Input: part model. Units: mm. Frame: model coordinates. A direction names the side the tool comes from. Give positions to 0.01 mm unless a question says otherwise; leave off trailing zeros. Order: outer loops, then holes, each group sorted by start corner. A loop starts at its lowest first (then second) coordinate and runs counter-clockwise, first axis right, second up. Notation, with made-up numbers: (-15, 44) -> (41, 44) arc R12 cw to (41, 66) -> close; hole circle Ø11 at (-38, 32). An arc over 180 degrees is marked (long way). Use a Markdown table: item, result. Add a question column.
from build123d import *

# Parameters (mm, degrees)
F1_DEPTH      = 25.4
F2_DEPTH      = 20.32
F3_SIZE2      = 12.7
F3_SIZE       = 25.4
F4_SIZE2      = 25.4
F4_SIZE       = 12.7
F4_2_SIZE2    = 25.4
F4_2_SIZE     = 12.7
F5_R          = 16.1148296274
F6_DEPTH      = 103.886
F8_DEPTH      = 109.4047297446
F8_DEPTH_BACK = 116.5023496438
F9_R          = 3.3795298113
F10_DEPTH     = 138.2457237613


with BuildPart() as f1:
    # F0 (on Top) → F1 (new body)
    with BuildSketch(Plane.XY):
        with BuildLine():
            ThreePointArc((52.5300336642, -32.2163809765), (59.3056389857, -16.7374079377), (61.6222333252, 0))
            ThreePointArc((61.6222333252, 0), (49.8558080108, 36.2173721792), (19.05, 58.6037297446))
            ThreePointArc((19.05, 58.6037297446), (0, 61.6222333252), (-19.05, 58.6037297446))
            ThreePointArc((-19.05, 58.6037297446), (-57.8186685482, 21.31434276), (-52.5300336642, -32.2163809765))
            ThreePointArc((-52.5300336642, -32.2163809765), (-39.9894732611, -46.8843435305), (-23.5270019404, -56.9541905366))
            ThreePointArc((-23.5270019404, -56.9541905366), (0, -61.6222333252), (23.5270019404, -56.9541905366))
            ThreePointArc((23.5270019404, -56.9541905366), (39.9894732611, -46.8843435305), (52.5300336642, -32.2163809765))
        make_face()
    extrude(amount=F1_DEPTH)

    # F0 (on Top) → F2 (join)
    with BuildSketch(Plane.XY):
        with BuildLine():
            ThreePointArc((-23.5270019404, -56.9541905366), (-39.9894732611, -46.8843435305), (-52.5300336642, -32.2163809765))
            Line((-52.5300336642, -32.2163809765), (-100.8460948708, -92.7285929554))
            Line((-100.8460948708, -92.7285929554), (-71.0725153171, -116.5013496438))
            Line((-71.0725153171, -116.5013496438), (-23.5270019404, -56.9541905366))
        make_face()
        with BuildLine():
            ThreePointArc((-19.05, 58.6037297446), (0, 61.6222333252), (19.05, 58.6037297446))
            Line((19.05, 58.6037297446), (19.05, 109.4037297446))
            Line((19.05, 109.4037297446), (-19.05, 109.4037297446))
            Line((-19.05, 109.4037297446), (-19.05, 58.6037297446))
        make_face()
        with BuildLine():
            Line((100.8460948708, -92.7285929554), (52.5300336642, -32.2163809765))
            ThreePointArc((52.5300336642, -32.2163809765), (39.9894732611, -46.8843435305), (23.5270019404, -56.9541905366))
            Line((23.5270019404, -56.9541905366), (71.0725153171, -116.5013496438))
            Line((71.0725153171, -116.5013496438), (100.8460948708, -92.7285929554))
        make_face()
    extrude(amount=F2_DEPTH)

    # F3
    f3_edges = [f1.edges().sort_by_distance(p)[0] for p in [
        (85.959305, -104.614971, 20.32),
    ]]
    f3_side = f1.faces().sort_by_distance((62.662137, -75.354715, 20.32))[0]
    chamfer(f3_edges, length=F3_SIZE, length2=F3_SIZE2, reference=f3_side)

    # F4
    f4_edges = [f1.edges().sort_by_distance(p)[0] for p in [
        (-85.959305, -104.614971, 20.32),
    ]]
    f4_side = f1.faces().sort_by_distance((-85.959305, -104.614971, 10.16))[0]
    chamfer(f4_edges, length=F4_SIZE, length2=F4_SIZE2, reference=f4_side)

    # F4#2
    f4_2_edges = [f1.edges().sort_by_distance(p)[0] for p in [
        (0, 109.40373, 20.32),
    ]]
    f4_2_side = f1.faces().sort_by_distance((0, 109.40373, 10.16))[0]
    chamfer(f4_2_edges, length=F4_2_SIZE, length2=F4_2_SIZE2, reference=f4_2_side)

    # F5 (on face) → F6 (join)
    with BuildSketch(Plane.XY.offset(25.4)):
        with Locations((-30.9876389802, 0)):
            Circle(F5_R)
        with Locations((30.9876389802, 0)):
            Circle(F5_R)
    extrude(amount=F6_DEPTH)

    # F7 (on Front) → F8 (cut, two sides)
    with BuildSketch(Plane.XZ) as f8_sk:
        Polygon((47.1024686075, 129.286), (37.3986288905, 129.286), (37.3986288905, 99.2526204783), (47.1024686075, 93.5718588345), align=None)
        Polygon((-47.1024686075, 129.286), (-47.1024686075, 93.5718588345), (-37.3986288905, 99.2526204783), (-37.3986288905, 129.286), align=None)
    extrude(amount=-F8_DEPTH, mode=Mode.SUBTRACT)
    extrude(f8_sk.sketch, amount=F8_DEPTH_BACK, mode=Mode.SUBTRACT)

    # F9 (on face) → F10 (cut, through all)
    with BuildSketch(Plane(origin=(-37.3986288905, 0, 0), x_dir=(0, -1, 0), z_dir=(-1, 0, 0))):
        with Locations((0, 124.0975558758)):
            Circle(F9_R)
    extrude(amount=-F10_DEPTH, mode=Mode.SUBTRACT)


solid = f1.part
Q1. Draft query along X for faces 4 (the cylindrical face through (-26.293, 0.733, 120.798)), 5 (the flat face through (-47.63, -87.14, 10.02)), 6 (the flat face through (-78.13, -94.39, 14.06)). Return one class per face: +X half, -X half, draft (parallel to the pull), parting line (faces both ways), or undercut.
Q2. Section query D-D (y = -40.5). Return loops of the section in (x, z).
Q3. Section query C-C (x = -31). Return loops of the section in (y, z).
Q4. Ray query, line 1 (Z direction, x = 25.25, y = 0); line 2 (Z direction, x = 56, y = 3); line 3 (X direction, y = -13.5, z = 108). Return the intervals inside material, ascending.
Q5. Section query B-B (z = 44.5). Return loops of the section in (x, y), plus the area to 3 significant figures.
Q6. First-contact query: pin 1 (3 mm diameter, centred on x = 28, z = 44, fed in from -Y); pin 2 (15 mm diameter, centred on y = 1.5, z = 121.5, fed in from -X); pin 3 (8 mm diameter, centred on x = -0.5, y = -19, fed in from +Z); pin 4 (6 mm diameter, centred on x = -17, y = 86, fed in from -Z). Flat tips, straight axial feed; report the tip coordinate or a pass-through.
Q7. Section query A-A (x = 0). Return loops of the section in (y, z).
Q8. Access query for faces 1 (the flat face through (-19.05, 79, 10)), 2 (the flat face through (19.05, 78, 10)), 3 (the flat face through (37.399, 0, 114)). Directions: +Z, -Z, +X, -X, +Y, -Y. A direction counts if a zero-diameter tool reaches every point of the face in a straight line with its end or side. Return the directions, or none.
Solution:
| question | item | result |
|---|---|---|
| 1 | face 4 | draft |
| 1 | face 5 | undercut |
| 1 | face 6 | -X half |
| 2 | outline | (-59.14, 0) -> (59.14, 0) -> (59.14, 20.32) -> (46.44, 20.32) -> (46.44, 25.4) -> (-46.44, 25.4) -> (-46.44, 20.32) -> (-59.14, 20.32) -> close |
| 3 | outline | (-66.31, 0) -> (53.26, 0) -> (53.26, 25.4) -> (16.11, 25.4) -> (16.11, 129.29) -> (-16.11, 129.29) -> (-16.11, 25.4) -> (-53.26, 25.4) -> (-53.26, 20.32) -> (-66.31, 20.32) -> close; hole circle Ø6.76 at (0, 124.1) |
| 4 | line 1 | z = 0 to 120.72, 127.48 to 129.29 |
| 4 | line 2 | z = 0 to 25.4 |
| 4 | line 3 | x = -37.4 to -22.19, 22.19 to 37.4 |
| 5 | outline | circle Ø32.23 at (-30.99, 0); circle Ø32.23 at (30.99, 0) |
| 5 | area | 1,630 mm² |
| 6 | pin 1 | stops at y = -16.05 |
| 6 | pin 2 | stops at x = -37.4 |
| 6 | pin 3 | stops at z = 25.4 |
| 6 | pin 4 | stops at z = 0 |
| 7 | outline | (-61.62, 0) -> (109.4, 0) -> (109.4, 7.62) -> (84, 20.32) -> (61.62, 20.32) -> (61.62, 25.4) -> (-61.62, 25.4) -> close |
| 8 | face 1 | +Z, -Z, -X, +Y |
| 8 | face 2 | +Z, -Z, +X, +Y |
| 8 | face 3 | +Z, +X, +Y, -Y |
